Answer from the drawing. Dimensions are ordinates in mm from the lowest x, y and z of the part. A direction names the side the tool comes from. Give positions to 0.01 mm unless a question says otherwise; leave off trailing zeros. Write each loop counter-clockwise with the first axis right and the second up, starting at its lowest first coordinate (ties: lowest second). Pieces come first, ordered by that corner, then holes. Notation, with made-up numbers: (-28, 58.25) -> (16, 58.25) arc R29 ccw to (16, 96.25) -> close; hole circle Ø3 at (-0.75, -40). An arc over 180 degrees is marked (long way). Use a Markdown table: item, result. Add a question column.
Q1. Section C-C, the plane y = 13 is taken. Give the vertices of the cut face in (x, z) (1 decimal), plus the area to 3 significant figures.
Q2. Section B-B, the plane y = 64 is taken. Give the vertices of the cut face in (x, z), plus the area to 3 significant figures.
Q3. For the marked faces 4, 5 and 6, determine the directions among +Z, -Z, +X, -X, +Y, -Y from which every point of the face is accessible in a straight line to the end or side of a thin tool.
Q4. Each of these flat-tipped pins is pushed along its axis until it touches: pin 1 Ø5 at (y, z) = (28.5, 50) entering from -X (1 decimal); pin 2 Ø8 at (y, z) = (48, 48) entering from -X; pin 3 Ø6 at (x, z) = (63.5, 76.5) entering from +Y (1 decimal). Where does it stop, or does it pass through?
Q5. Consider line 1 (Z direction, x = 60, y = 23); line 2 (Z direction, x = 13, y = 16.5) (1 decimal); line 3 (Z direction, x = 3.5, y = 31.5). Determine where each line is inside the solid, lowest interval first.
Q6. For a pull along Z with two mould halves and no side action, classify the marked faces 1, 2 and 3 as pulls with the +Z half, pulls with the -Z half, needs draft (parallel to the pull), parting line crosses it, or undercut.
Q7. Section D-D, the plane z = 22.5 is taken. Give the vertices of the cut face in (x, y), plus the area to 3 significant figures.
Q8. Section A-A, the plane x = 63 is taken. Give the vertices of the cut face in (y, z) (1 decimal), plus the area to 3 significant figures.
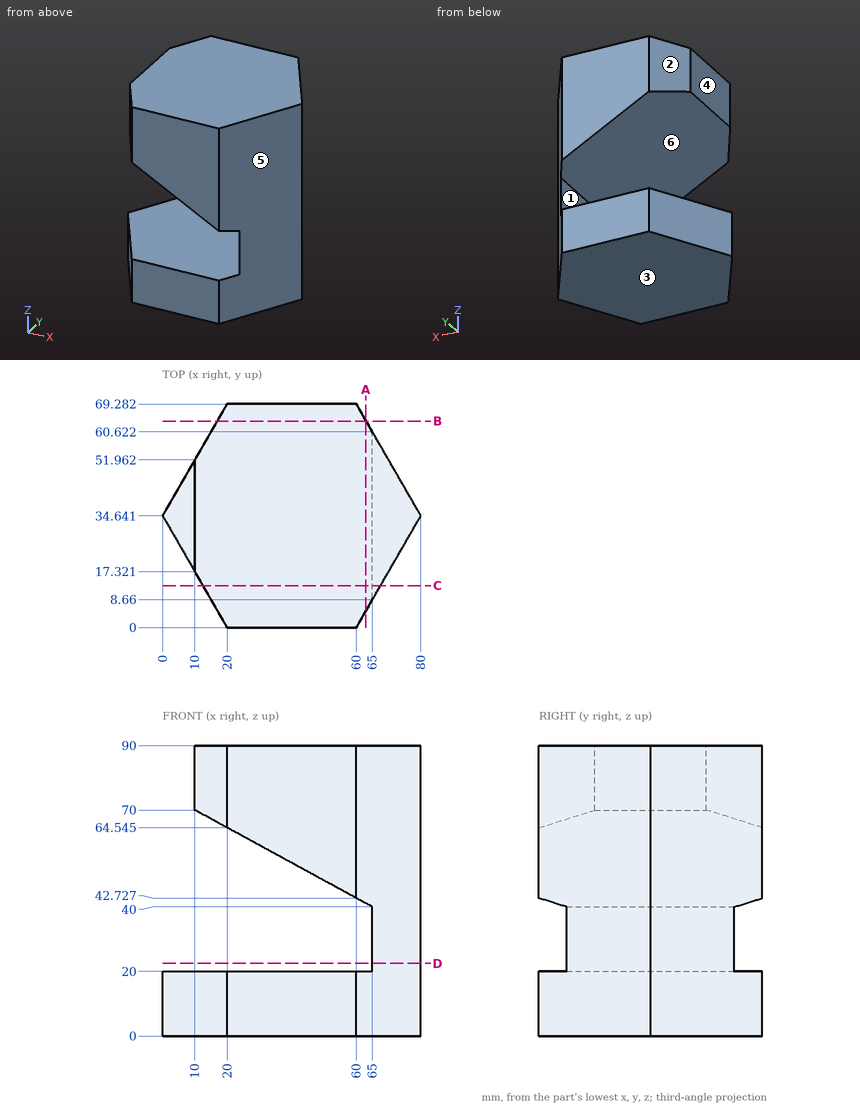
Result set:
| question | item | result |
|---|---|---|
| 1 | outline | (12.5, 0) -> (67.5, 0) -> (67.5, 90) -> (12.5, 90) -> (12.5, 68.6) -> (65, 40) -> (65, 20) -> (12.5, 20) -> close |
| 1 | area | 3,150 mm2 |
| 2 | outline | (16.95, 0) -> (63.05, 0) -> (63.05, 20) -> (16.95, 20) -> close; (16.95, 66.21) -> (63.05, 41.06) -> (63.05, 90) -> (16.95, 90) -> close |
| 2 | area | 2,600 mm2 |
| 3 | face 4 | +Z, -X, +Y, -Y |
| 3 | face 5 | +Z, -Z, +X, -Y |
| 3 | face 6 | -X, +Y, -Y |
| 4 | pin 1 | stops at x = 42.1 |
| 4 | pin 2 | stops at x = 43 |
| 4 | pin 3 | stops at y = 68.4 |
| 5 | line 1 | z = 0 to 20, 42.73 to 90 |
| 5 | line 2 | z = 0 to 20, 68.4 to 90 |
| 5 | line 3 | z = 0 to 20 |
| 6 | face 1 | undercut |
| 6 | face 2 | needs draft |
| 6 | face 3 | pulls with the -Z half |
| 7 | outline | (65, 8.66) -> (80, 34.64) -> (65, 60.62) -> close |
| 7 | area | 390 mm2 |
| 8 | outline | (5.2, 0) -> (64.1, 0) -> (64.1, 20) -> (5.2, 20) -> close; (5.2, 41.1) -> (64.1, 41.1) -> (64.1, 90) -> (5.2, 90) -> close |
| 8 | area | 4,060 mm2 |
